from build123d import *

# Parameters (mm, degrees)
SKETCH1_R           = 5
BOSS_EXTRUDE1_DEPTH = 8
FILLET1_R           = 0.125
SKETCH4_R           = 2
CUT_EXTRUDE1_DEPTH  = 2.5


with BuildPart() as part:
    # Sketch1 → Boss-Extrude1 (new body)
    with BuildSketch(Plane.XY):
        Circle(SKETCH1_R)
        with BuildLine():
            ThreePointArc((0.5, -1.75), (2.25, 0), (0.5, 1.75))
            Line((0.5, 1.75), (-0.5402042, 1.75))
            ThreePointArc((-0.5402042, 1.75), (-2.2902042, 0), (-0.5402042, -1.75))
            Line((-0.5402042, -1.75), (0.5, -1.75))
        make_face(mode=Mode.SUBTRACT)
    extrude(amount=BOSS_EXTRUDE1_DEPTH)

    # Fillet1
    fillet1_edges = [part.edges().sort_by_distance(p)[0] for p in [
        (-5, 0, 8),
        (-5, 0, 0),
    ]]
    fillet(fillet1_edges, radius=FILLET1_R)

    # Sketch4 → Cut-Extrude1 (cut)
    with BuildSketch(Plane.XZ.offset(5)):
        with Locations((0, 4)):
            Circle(SKETCH4_R)
    extrude(amount=-CUT_EXTRUDE1_DEPTH, mode=Mode.SUBTRACT)


solid = part.part
CAD build for the part. Positions are in the model's coordinates, mm. A direction names the side the tool comes from. Give positions to 0.01 mm unless a question says otherwise; leave off trailing zeros. Order: outer loops, then holes, each group sorted by start corner. A loop starts at its lowest first (then second) coordinate and runs counter-clockwise, first axis right, second up. Notation, with made-up numbers: (71, -31) - (100, -31) arc R26 cw to (100, -3) - close; hole circle Ø4 at (-17.5, -20). An arc over 180 degrees is marked (long way). Write each question's results on one line, items separated by ' | '.
1. Saw through at A-A on x = 0. List the corners of the cut face in (y, z) (3 decimals).
Calculated:
outline: (-5, 0.125) arc R0.125 ccw to (-4.875, 0) - (-1.75, 0) - (-1.75, 8) - (-4.875, 8) arc R0.125 ccw to (-5, 7.875) - (-5, 6) - (-2.5, 6) - (-2.5, 2) - (-5, 2) - close; (1.75, 0) - (4.875, 0) arc R0.125 ccw to (5, 0.125) - (5, 7.875) arc R0.125 ccw to (4.875, 8) - (1.75, 8) - close
2. Pin check, flat tips, straight feed: pin 1 (1 mm diameter, centred on x = -3.5, z = 5.5, fed in from +Y); pin 2 (1 mm diameter, centred on y = 1.5, z = 5.5, fed in from -X); pin 3 (2 mm diameter, centred on y = -2.5, z = 2.5, fed in from +X). Stop position of each tip, or through.
Calculated:
pin 1: stops at y = 4 | pin 2: stops at x = -4.9 | pin 3: stops at x = 4.77
3. Pull direction X, two halves, no side cores. Call faces 4 (the face through (0, -1.75, 4)), 5 (the face through (3, 4, 4)), 6 (the face through (0, -2, 0)), 7 (the face through (2.25, -0.04, 3.94)): released by +X, released by -X, zero draft, split by the parting line, or undercut.
Calculated:
face 4: undercut | face 5: split by the parting line | face 6: zero draft | face 7: undercut
4. Probe L1, parallel to Z at x = 0, y = -4.3; L2, parallel to Y at x = 0, z = 5.25; L3, parallel to X at y = -3.4, z = 4. List the from-to ranges inside material, lowest first. Write a range as from..to.
Calculated:
L1: z = 0..2, 6..8 | L2: y = -2.5..-1.75, 1.75..5 | L3: x = -3.67..-2, 2..3.67
5. Saw through at B-B on y = 0. List the corners of the cut face in (x, z) (3 decimals).
Calculated:
outline: (-5, 0.125) arc R0.125 ccw to (-4.875, 0) - (-2.29, 0) - (-2.29, 8) - (-4.875, 8) arc R0.125 ccw to (-5, 7.875) - close; (2.25, 0) - (4.875, 0) arc R0.125 ccw to (5, 0.125) - (5, 7.875) arc R0.125 ccw to (4.875, 8) - (2.25, 8) - close
6. Saw through at C-C on z = 7. List the corners of the cut face in (x, y).
Calculated:
outline: circle Ø10 at (0, 0); hole (-0.54, -1.75) - (0.5, -1.75) arc R1.75 ccw to (0.5, 1.75) - (-0.54, 1.75) arc R1.75 ccw to start
7. 3-axis set-ups, long thin cutter, end or side, ignore diameter. For faces 1 (the face through (0, -2, 8)), 2 (the face through (-2.29, 0.04, 3.94)), 3 (the face through (1.847, -3.768, 3.234)): which of +Z, -Z, +X, -X, +Y, -Y reach the whole face in a straight line?
Calculated:
face 1: +Z, +X, -X, +Y, -Y | face 2: +Z, -Z | face 3: -Y
8. Saw through at D-D on z = 5.75. List the corners of the cut face in (x, y), and give its area (3 significant figures).
Calculated:
outline: (-0.97, -4.91) - (-0.97, -2.5) - (0.97, -2.5) - (0.97, -4.91) arc R5 ccw (long way) to start; hole (-0.54, -1.75) - (0.5, -1.75) arc R1.75 ccw to (0.5, 1.75) - (-0.54, 1.75) arc R1.75 ccw to start | area: 60.5 mm2
